from build123d import *

# Parameters (mm, degrees)
FORO_PER_VITE_M5_1_D           = 5.5
FORO_PER_VITE_M5_1_DEPTH       = 15.347633298
FORO_PER_VITE_M5_1_CSINK_D     = 5.55
FORO_PER_VITE_M5_1_CSINK_ANGLE = 90
FORO_PER_VITE_M5_1_TIP         = 1.652366702


with BuildPart() as part:
    # Schizzo1 → Rivoluzione1 (revolve)
    with BuildSketch(Plane.XY, mode=Mode.PRIVATE) as rivoluzione1_sk:
        Polygon((-152.5, 0), (152.5, 0), (152.5, 61.5), (87.5, 61.5), (87.5, 70), (80.5, 70), (80.5, 40), (35.5, 40), (35.5, 70), (28.5, 70), (28.5, 101), (-44.5, 101), (-44.5, 61.5), (-152.5, 61.5), align=None)
    revolve(rivoluzione1_sk.sketch.rotate(Axis((-1716.324322208, 0, 0), (1, 0, 0)), 90), axis=Axis((-1716.324322208, 0, 0), (1, 0, 0)))

    # Foro per Vite M5-1
    with Locations(Plane(origin=(-44.5, 96, 0), x_dir=(0, 0, -1), z_dir=(-1, 0, 0))):
        with Locations((0, 0), (-96, 96), (0, 192), (96, 96)):
            CounterSinkHole(FORO_PER_VITE_M5_1_D / 2, FORO_PER_VITE_M5_1_CSINK_D / 2, depth=FORO_PER_VITE_M5_1_DEPTH, counter_sink_angle=FORO_PER_VITE_M5_1_CSINK_ANGLE)
            with Locations((0, 0, -(FORO_PER_VITE_M5_1_DEPTH + FORO_PER_VITE_M5_1_TIP / 2))):  # 118° drill point
                Cone(0, FORO_PER_VITE_M5_1_D / 2, FORO_PER_VITE_M5_1_TIP, mode=Mode.SUBTRACT)


solid = part.part
Here's how the part is built. I have some questions about the finished solid (model axes, mm). A direction names the side the tool comes from. Coordinates: 2 decimals unless noted, no trailing zeros. Write each loop counter-clockwise with the first axis right and the second up, starting at its lowest first coordinate (ties: lowest second). Pieces come first, ordered by that corner, then holes.
1) Thinking about a two-plate mould opening in X: for faces 1 (the face through (-44.5, 43, -46)), 2 (the face through (80.5, 30, 30)), 3 (the face through (119.545, -60.977, -8.006)), which applies, +X half, -X half, draft (parallel to the pull), parting line (faces both ways), or undercut?
Filled in:
face 1: -X half
face 2: undercut
face 3: draft
2) If we section it at A-A (z = 44): List the corners of the cut face in (x, y) for me.
Filled in:
outline: (-152.5, -42.97) - (-44.5, -42.97) - (-44.5, -90.91) - (28.5, -90.91) - (28.5, -54.44) - (35.5, -54.44) - (35.5, 54.44) - (28.5, 54.44) - (28.5, 90.91) - (-44.5, 90.91) - (-44.5, 42.97) - (-152.5, 42.97) - close; (80.5, -54.44) - (87.5, -54.44) - (87.5, -42.97) - (152.5, -42.97) - (152.5, 42.97) - (87.5, 42.97) - (87.5, 54.44) - (80.5, 54.44) - close
3) If we section it at C-C (x = -95): List the corners of the cut face in (y, z) for me.
Filled in:
outline: circle Ø123 at (0, 0)
4) If I drill on line 1 (Y direction, x = -34.75, z = 0); line 2 (X direction, y = -7.5, z = -46); line 3 (X direction, y = 62.5, z = -55), over which ranges is the centre line in solid material (lowest first)?
Filled in:
line 1: y = -101 to -98.75, -93.25 to 93.25, 98.75 to 101
line 2: x = -152.5 to 35.5, 80.5 to 152.5
line 3: x = -44.5 to 28.5
5) Which directions (+Z, -Z, +X, -X, +Y, -Y) give clear straight access to the entire face, cutting with the end or side of a thin tool? Please do faces 4 (the face through (31.951, 68.335, -15.175)), 5 (the face through (57.68, -1.76, -39.96)), 6 (the face through (-152.5, -1, -1)), 7 (the face through (-99.256, -60.977, -8.006)).
Filled in:
face 4: +X
face 5: none
face 6: +Z, -Z, -X, +Y, -Y
face 7: -X
6) If we section it at B-B (y = -33): List the corners of the cut face in (x, z) for me, plus the area to 3 significant figures.
Filled in:
outline: (-152.5, -51.9) - (-44.5, -51.9) - (-44.5, -95.46) - (28.5, -95.46) - (28.5, -61.73) - (35.5, -61.73) - (35.5, -22.61) - (80.5, -22.61) - (80.5, -61.73) - (87.5, -61.73) - (87.5, -51.9) - (152.5, -51.9) - (152.5, 51.9) - (87.5, 51.9) - (87.5, 61.73) - (80.5, 61.73) - (80.5, 22.61) - (35.5, 22.61) - (35.5, 61.73) - (28.5, 61.73) - (28.5, 95.46) - (-44.5, 95.46) - (-44.5, 51.9) - (-152.5, 51.9) - close
area: 35,700 mm2
7) If we section it at D-D (z = 78): List the corners of the cut face in (x, y) for me, plus the area to 3 significant figures.
Filled in:
outline: (-44.5, -64.16) - (28.5, -64.16) - (28.5, 64.16) - (-44.5, 64.16) - close
area: 9,370 mm2
8) I'm going to push flat-ended pins straight in: pin 1 (3.5 mm diameter, centred on y = 0, z = -96, fed in from -X); pin 2 (1.5 mm diameter, centred on x = -59.5, z = -10.5, fed in from +Y); pin 3 (1.5 mm diameter, centred on x = -11, y = 29, fed in from -Z). Where does each tip first touch, or does it pass through?
Filled in:
pin 1: stops at x = -28.55
pin 2: stops at y = 60.72
pin 3: stops at z = -96.97
